Model file for the job. Use its own axes, mm. Round coordinates to 2 decimals unless told otherwise and drop trailing zeros. Loops run counter-clockwise (first coordinate to the right, second up) from the corner with the lowest first, then second, coordinate; pieces in that order, holes last. Notation, with made-up numbers: M 78,85.25 L 101,85.25 A8 ccw 101,100.25 Z; hole C 42,62 d6. An arc over 180 degrees is marked long. Use a Markdown table: item, result. Add a question column.
Item 1: Saw through at C-C on y = 10.75. Give the number of separate pieces and of enclosed holes in the cut face, then the cut area to 3 significant figures.
Item 2: Two-plate mould, pull along X, no slides. Class faces 1 (the cylindrical face through (-2.136, 15.756, -0.488)), 2 (the flat face through (0, 0, 0)), 3 (the cylindrical face through (4.84, 12.32, 15.38)): +X half, -X half, draft (parallel to the pull), parting line (faces both ways), or undercut.
Item 3: Saw through at D-D on y = 4.75. Write the cut outline in (x, z) (3 decimals).
Item 4: Saw through at A-A on x = 0. Write the cut outline in (y, z) (3 decimals), then the cut area to 3 significant figures.
Item 5: Pin check, flat tips, straight feed: P1, Ø1, axis at x = -12, y = 11, coming from the -Z side; P2, Ø12, axis at x = 8, y = 5.5, coming from the -Z side; P3, Ø2.5, axis at x = 9.5, z = 2.5, coming from the +Y side; P4, Ø8, axis at x = -9.03, z = 7.84, coming from the +Y side. Stop position of each tip, or through.
Item 6: Saw through at B-B on z = -11.5. Write the cut outline in (x, y).
Item 7: Wall check: L1, parallel to Y at x = -9.5, z = -5.5; L2, parallel to X at y = 14.5, z = 4.5; L3, parallel to X at y = 10.25, z = 7. Give the ranges that are in metal, low to high. Write a range as from..to.
```python
from build123d import *

# Parameters (mm, degrees)
SKETCH1_R           = 16.125
BOSS_EXTRUDE1_DEPTH = 25
SKETCH2_R           = 2.45
CUT_EXTRUDE1_DEPTH  = 18.75
SKETCH3_R           = 2.45
CUT_EXTRUDE2_DEPTH  = 18.75
SKETCH4_R           = 2.45
CUT_EXTRUDE3_DEPTH  = 18.75
SKETCH5_R           = 2.45
CUT_EXTRUDE5_DEPTH  = 18.75


with BuildPart() as part:
    # Sketch1 → Boss-Extrude1 (new body)
    with BuildSketch(Plane(origin=(0, 0, 0), x_dir=(1, 0, 0), z_dir=(0, 1, 0))):
        with Locations(Location((0, 0, 0), (0, 0, 270))):
            Circle(SKETCH1_R)
    extrude(amount=BOSS_EXTRUDE1_DEPTH)

    # Sketch2 → Cut-Extrude1 (cut)
    with BuildSketch(Plane(origin=(0, 25, 0), x_dir=(1, 0, 0), z_dir=(0, 1, 0))):
        with Locations(Location((0, -2.6, 0), (0, 0, 270))):
            Circle(SKETCH2_R)
        with Locations(Location((0, 2.6, 0), (0, 0, 270))):
            Circle(SKETCH2_R)
        with Locations(Location((0, 7.8, 0), (0, 0, 270))):
            Circle(SKETCH2_R)
        with Locations(Location((0, 13, 0), (0, 0, 270))):
            Circle(SKETCH2_R)
        with Locations(Location((0, -7.8, 0), (0, 0, 270))):
            Circle(SKETCH2_R)
        with Locations(Location((0, -13, 0), (0, 0, 270))):
            Circle(SKETCH2_R)
    extrude(amount=-CUT_EXTRUDE1_DEPTH, mode=Mode.SUBTRACT)

    # Sketch3 → Cut-Extrude2 (cut)
    with BuildSketch(Plane(origin=(0, 25, 0), x_dir=(1, 0, 0), z_dir=(0, 1, 0))):
        with Locations(Location((4.528018354, -0.043234507, 0), (0, 0, 270))):
            Circle(SKETCH3_R)
        with Locations(Location((4.528018354, 5.156765493, 0), (0, 0, 270))):
            Circle(SKETCH3_R)
        with Locations(Location((4.528018354, -5.243234507, 0), (0, 0, 270))):
            Circle(SKETCH3_R)
        with Locations(Location((4.528018354, -10.443234507, 0), (0, 0, 270))):
            Circle(SKETCH3_R)
        with Locations(Location((4.528018354, 10.356765493, 0), (0, 0, 270))):
            Circle(SKETCH3_R)
    cut_extrude2 = extrude(amount=-CUT_EXTRUDE2_DEPTH, mode=Mode.SUBTRACT)

    # Sketch4 → Cut-Extrude3 (cut)
    with BuildSketch(Plane(origin=(0, 25, 0), x_dir=(1, 0, 0), z_dir=(0, 1, 0))):
        with Locations(Location((9.031350453, 7.756765493, 0), (0, 0, 270))):
            Circle(SKETCH4_R)
        with Locations(Location((9.031350453, 2.556765493, 0), (0, 0, 270))):
            Circle(SKETCH4_R)
        with Locations(Location((9.031350453, -2.643234507, 0), (0, 0, 270))):
            Circle(SKETCH4_R)
        with Locations(Location((9.031350453, -7.843234507, 0), (0, 0, 270))):
            Circle(SKETCH4_R)
    cut_extrude3 = extrude(amount=-CUT_EXTRUDE3_DEPTH, mode=Mode.SUBTRACT)

    # Sketch5 → Cut-Extrude5 (cut)
    with BuildSketch(Plane(origin=(0, 25, 0), x_dir=(1, 0, 0), z_dir=(0, 1, 0))):
        with Locations(Location((13.534682553, -0.043234507, 0), (0, 0, 270))):
            Circle(SKETCH5_R)
    cut_extrude5 = extrude(amount=-CUT_EXTRUDE5_DEPTH, mode=Mode.SUBTRACT)

    # Mirror2: Cut-Extrude2, Cut-Extrude3, Cut-Extrude5 across plane
    add(cut_extrude2.mirror(Plane(origin=(0, 0, 0), x_dir=(0, 0, 1), z_dir=(1, 0, 0))), mode=Mode.SUBTRACT)
    add(cut_extrude3.mirror(Plane(origin=(0, 0, 0), x_dir=(0, 0, 1), z_dir=(1, 0, 0))), mode=Mode.SUBTRACT)
    add(cut_extrude5.mirror(Plane(origin=(0, 0, 0), x_dir=(0, 0, 1), z_dir=(1, 0, 0))), mode=Mode.SUBTRACT)


solid = part.part
```
Entries:
| question | item | result |
|---|---|---|
| 1 | separate pieces | 1 |
| 1 | enclosed holes | 26 |
| 1 | area | 327 mm2 |
| 2 | face 1 | undercut |
| 2 | face 2 | draft |
| 2 | face 3 | parting line |
| 3 | outline | C 0,0 d32.25 |
| 4 | outline | M 0,-16.125 L 25,-16.125 L 25,-15.45 L 6.25,-15.45 L 6.25,-10.55 L 25,-10.55 L 25,-10.25 L 6.25,-10.25 L 6.25,-5.35 L 25,-5.35 L 25,-5.05 L 6.25,-5.05 L 6.25,-0.15 L 25,-0.15 L 25,0.15 L 6.25,0.15 L 6.25,5.05 L 25,5.05 L 25,5.35 L 6.25,5.35 L 6.25,10.25 L 25,10.25 L 25,10.55 L 6.25,10.55 L 6.25,15.45 L 25,15.45 L 25,16.125 L 0,16.125 Z |
| 4 | area | 255 mm2 |
| 5 | P1 | z = -11.3 |
| 5 | P2 | z = -16 |
| 5 | P3 | y = 6.25 |
| 5 | P4 | y = 25 |
| 6 | outline | M -11.3,0 L 11.3,0 L 11.3,25 L 6.69,25 L 6.69,6.25 L 2.36,6.25 L 2.36,25 L 1.94,25 L 1.94,6.25 L -1.94,6.25 L -1.94,25 L -2.36,25 L -2.36,6.25 L -6.69,6.25 L -6.69,25 L -11.3,25 Z |
| 7 | L1 | 0..6.25 |
| 7 | L2 | -15.48..-10.63, -7.43..-6.86, -2.19..-1.55, 1.55..2.19, 6.86..7.43, 10.63..15.48 |
| 7 | L3 | -14.53..-11.33, -6.73..-6.24, -2.82..-2.32, 2.32..2.82, 6.24..6.73, 11.33..14.53 |
